```python
from build123d import *

# Parameters (mm, degrees)
F1_DEPTH = 25.4
F2_SIZE  = 1.016
F3_W     = 3
F3_H     = 19.05
F4_DEPTH = 25.4
F5_W     = 5.08
F5_H     = 5.08
F5_W_2   = 1.27
F5_H_2   = 1.27
F6_DEPTH = 6.501
F7_R     = 2.5


with BuildPart() as f1:
    # F0 (on Top) → F1 (new body)
    with BuildSketch(Plane.XY):
        with BuildLine():
            Line((0.635, 15.1509385957), (0.635, 2.4509385957))
            ThreePointArc((0.635, 2.4509385957), (5.0286441204, -1.3802173742), (-0.635, 0))
            Line((-0.635, 0), (-0.635, 15.1509385957))
            Line((-0.635, 15.1509385957), (-2.635, 15.1509385957))
            Line((-2.635, 15.1509385957), (-2.635, 0))
            ThreePointArc((-2.635, 0), (5.8037497728, -3.6297382826), (2.635, 4.9927046778))
            Line((2.635, 4.9927046778), (2.635, 15.1509385957))
            Line((2.635, 15.1509385957), (0.635, 15.1509385957))
        make_face()
    extrude(amount=F1_DEPTH)

    # F2
    f2_edges = [f1.edges().sort_by_distance(p)[0] for p in [
        (-0.635, 15.150939, 12.7),
        (0.635, 15.150939, 12.7),
    ]]
    chamfer(f2_edges, length=F2_SIZE)

    # F3 (on Top) → F4 (join, through all)
    with BuildSketch(Plane.XY):
        with Locations((2.365, -14.2946960071)):
            Rectangle(F3_W, F3_H)
    extrude(amount=F4_DEPTH)

    # F5 (on face) → F6 (cut, through all)
    with BuildSketch(Plane.YZ.offset(3.865)):
        with Locations((-7.3096960071, 5.08)):
            Rectangle(F5_W, F5_H)
        with Locations((-17.4696960071, 12.7)):
            Rectangle(F5_W, F5_H)
        with Locations((-23.1846960071, 5.08)):
            Rectangle(F5_W_2, F5_H)
        with Locations((-17.4696960071, 24.765)):
            Rectangle(F5_W, F5_H_2)
    extrude(amount=-F6_DEPTH, mode=Mode.SUBTRACT)

    # F7
    f7_edges = [f1.edges().sort_by_distance(p)[0] for p in [
        (0.635, 2.450939, 12.7),
        (-2.635, 0, 12.7),
        (2.635, 4.992705, 12.7),
        (3.865, -4.769696, 16.51),
        (0.865, -4.769696, 16.51),
        (0.865, -4.769696, 1.27),
        (3.865, -4.769696, 1.27),
    ]]
    fillet(f7_edges, radius=F7_R)


solid = f1.part
```
Source: CAD feature listing. Evaluate the final solid. Frame: model axes, mm. A direction names the side the tool comes from. Coordinates: 2 decimals unless noted, no trailing zeros. Loops run counter-clockwise (first coordinate to the right, second up) from the corner with the lowest first, then second, coordinate; pieces in that order, holes last. Notation, with made-up numbers: M 0.5,54.5 L 53.5,54.5 A21 cw 53.5,93.5 Z; hole C 58.25,53.25 d10. An arc over 180 degrees is marked long. Use a Markdown table: item, result. Add a question column.
Q1. Section query D-D, the plane z = 6.25. Return loops of the section in (x, y) (3 decimals).
Q2. Section query A-A, the plane y = -15.5. Return loops of the section in (x, z) (3 decimals).
Q3. Section query B-B, the plane z = 14. Return loops of the section in (x, y) (3 decimals).
Q4. Section query C-C, the plane y = 12.5. Return loops of the section in (x, z) (3 decimals).
Q5. Material intervals for L1, parallel to Z at x = 3.25, y = -15.5; L2, parallel to X at y = 10, z = 20 (3 decimals); L3, parallel to X at y = -7, z = 11.5 (3 decimals), sorted ascending.
Q6. Draft query along Z for faces 1 (the flat face through (-1, 0, 25.4)), 2 (the flat face through (2, -14.93, 25)), 3 (the flat face through (2, -20.01, 13)). Return one class per face: pulls with the +Z half, pulls with the -Z half, needs draft (parallel to the pull), parting line crosses it, or undercut.
Q7. Access query for faces 4 (the flat face through (-0.635, 7, 13)), 5 (the cylindrical face through (1.231, 3.825, 12.878)), 6 (the flat face through (2, -20.01, 25)), 7 (the flat face through (2, -23, 7.62)). Directions: +Z, -Z, +X, -X, +Y, -Y. A direction counts if a zero-diameter tool reaches every point of the face in a straight line with its end or side. Return the directions, or none.
Q8. First-contact query: pin 1 (1.5 mm diameter, centred on x = 2.5, y = -17.5, fed in from +Z); pin 2 (14 mm diameter, centred on y = -18, z = 15.5, fed in from +X) (3 decimals); pin 3 (1.5 mm diameter, centred on x = 4, z = 3.5, fed in from -Y); pin 4 (5.5 mm diameter, centred on x = 2.365, y = 0, fed in from +Z). Flat tips, straight axial feed; report the tip coordinate or a pass-through.
Result:
| question | item | result |
|---|---|---|
| 1 | outline | M -2.635,0 A5 ccw 0.865,-4.77 L 3.865,-4.77 A5 ccw 4.212,4.646 A2.5 cw 2.635,6.97 L 2.635,15.151 L 1.651,15.151 L 0.635,14.135 L 0.635,5.446 A2.5 ccw 2.785,2.97 A3 cw long -0.635,0 L -0.635,14.135 L -1.651,15.151 L -2.635,15.151 Z; M 0.865,-22.55 L 3.865,-22.55 L 3.865,-9.85 L 0.865,-9.85 Z |
| 2 | outline | M 0.865,0 L 3.865,0 L 3.865,10.16 L 0.865,10.16 Z; M 0.865,15.24 L 3.865,15.24 L 3.865,24.13 L 0.865,24.13 Z |
| 3 | outline | M -2.635,0 A5 ccw -0.302,-4.23 A2.5 cw 0.865,-6.344 L 0.865,-14.93 L 3.865,-14.93 L 3.865,-6.344 A2.5 cw 5.032,-4.23 A5 ccw 4.212,4.646 A2.5 cw 2.635,6.97 L 2.635,15.151 L 1.651,15.151 L 0.635,14.135 L 0.635,5.446 A2.5 ccw 2.785,2.97 A3 cw long -0.635,0 L -0.635,14.135 L -1.651,15.151 L -2.635,15.151 Z; M 0.865,-23.82 L 3.865,-23.82 L 3.865,-20.01 L 0.865,-20.01 Z |
| 4 | outline | M -2.635,0 L -0.635,0 L -0.635,25.4 L -2.635,25.4 Z; M 0.635,0 L 2.635,0 L 2.635,25.4 L 0.635,25.4 Z |
| 5 | L1 | z = 0 to 10.16, 15.24 to 24.13 |
| 5 | L2 | x = -2.635 to -0.635, 0.635 to 2.635 |
| 5 | L3 | x = 0.865 to 3.865 |
| 6 | face 1 | pulls with the +Z half |
| 6 | face 2 | needs draft |
| 6 | face 3 | undercut |
| 7 | face 4 | +Z, -Z, +Y |
| 7 | face 5 | +Z, -Z |
| 7 | face 6 | +Z, +X, -X |
| 7 | face 7 | +X, -X, -Y |
| 8 | pin 1 | stops at z = 24.13 |
| 8 | pin 2 | stops at x = 3.865 |
| 8 | pin 3 | stops at y = -22.55 |
| 8 | pin 4 | passes through |
